Geometry check sheet. Reference: drawing and pictorial views, mm from the part's lowest x, y, z. A direction names the side the tool comes from. Round coordinates to 2 decimals unless told otherwise and drop trailing zeros. Loops run counter-clockwise (first coordinate to the right, second up) from the corner with the lowest first, then second, coordinate; pieces in that order, holes last. Notation, with made-up numbers: (17.5, -39.75) -> (31.5, -39.75) arc R17 ccw to (31.5, -17.75) -> close; hole circle Ø9 at (70.25, 3). An arc over 180 degrees is marked (long way). Use one line per item in the form item = value.
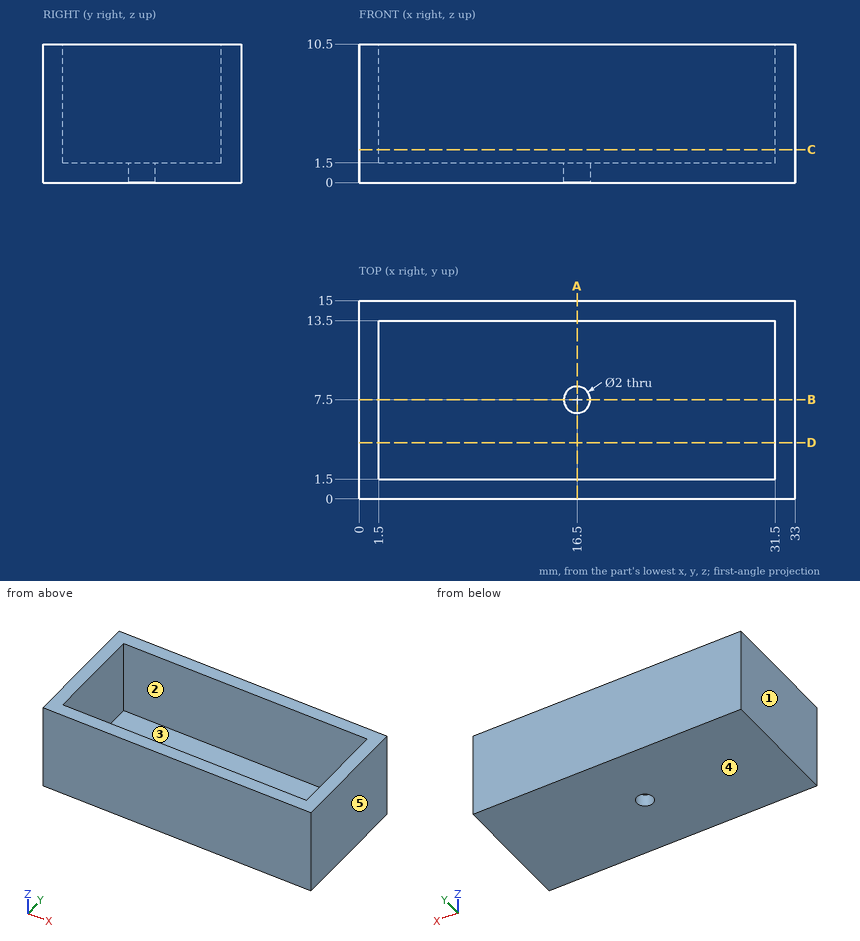
1. Mould release check, pull along X, two halves, no side actions. Record for the marked faces 3, 4 and 5: released by +X, released by -X, zero draft, split by the parting line, or undercut.
Return value:
face_3 = undercut
face_4 = zero draft
face_5 = released by +X
2. Gauge pin test, flat ends, axial feed: pin 1 (1 mm diameter, centred on y = 5.5, z = 2.5, fed in from -X); pin 2 (3.5 mm diameter, centred on x = 20, y = 9.5, fed in from +Z). Record the tip position at first contact, or that the pin passes through.
Return value:
pin_1 = 0
pin_2 = 1.5
3. Section check B-B (y = 7.5). Record the boundary of the cut face in (x, z), then the cut area to 3 significant figures.
Return value:
outline = (0, 0) -> (15.5, 0) -> (15.5, 1.5) -> (1.5, 1.5) -> (1.5, 10.5) -> (0, 10.5) -> close; (17.5, 0) -> (33, 0) -> (33, 10.5) -> (31.5, 10.5) -> (31.5, 1.5) -> (17.5, 1.5) -> close
area = 73.5 mm2
4. Section check C-C (z = 2.5). Record the boundary of the cut face in (x, y), then the cut area to 3 significant figures.
Return value:
outline = (0, 0) -> (33, 0) -> (33, 15) -> (0, 15) -> close; hole (1.5, 1.5) -> (31.5, 1.5) -> (31.5, 13.5) -> (1.5, 13.5) -> close
area = 135 mm2
5. Section check D-D (y = 4.25). Record the boundary of the cut face in (x, z), then the cut area to 3 significant figures.
Return value:
outline = (0, 0) -> (33, 0) -> (33, 10.5) -> (31.5, 10.5) -> (31.5, 1.5) -> (1.5, 1.5) -> (1.5, 10.5) -> (0, 10.5) -> close
area = 76.5 mm2
6. Section check A-A (x = 16.5). Record the boundary of the cut face in (y, z).
Return value:
outline = (0, 0) -> (6.5, 0) -> (6.5, 1.5) -> (1.5, 1.5) -> (1.5, 10.5) -> (0, 10.5) -> close; (8.5, 0) -> (15, 0) -> (15, 10.5) -> (13.5, 10.5) -> (13.5, 1.5) -> (8.5, 1.5) -> close
7. Tool access check on the marked faces 1 and 2. Record the directions out of +Z, -Z, +X, -X, +Y, -Y that give a thin tool (end or side, any length) a straight path to the whole face; none if there is none.
Return value:
face_1 = +Z, -Z, -X, +Y, -Y
face_2 = +Z
8. Material ranges on line 1 along X through (y, z) = (7, 8.5); line 2 along Y through (x, z) = (16.5, 0.7); line 3 along Y through (x, z) = (7, 7.25), recorded low to high.
Return value:
line_1 = 0 to 1.5, 31.5 to 33
line_2 = 0 to 6.5, 8.5 to 15
line_3 = 0 to 1.5, 13.5 to 15
